```python
from build123d import *

# Parameters (mm, degrees)
BOSS_EXTRUDE1_DEPTH = 304.8
SHELL1_T            = -12.7


with BuildPart() as part:
    # Sketch1 → Boss-Extrude1 (new body)
    with BuildSketch(Plane(origin=(0, 0, 0), x_dir=(0, 0, -1), z_dir=(1, 0, 0))):
        Polygon((0, 0), (304.8, 0), (304.8, 56), (0, 109.74446372), align=None)
    extrude(amount=BOSS_EXTRUDE1_DEPTH)

    # Shell1
    shell1_openings = [part.faces().sort_by_distance(p)[0] for p in [
        (152.4, 82.87223186, -152.4),
    ]]
    offset(amount=SHELL1_T, openings=shell1_openings, kind=Kind.INTERSECTION)


solid = part.part
```
CAD build for the part. Positions are in the model's coordinates, mm. A direction names the side the tool comes from. Round coordinates to 2 decimals unless told otherwise and drop trailing zeros. Write each loop counter-clockwise with the first axis right and the second up, starting at its lowest first coordinate (ties: lowest second). Pieces come first, ordered by that corner, then holes. Notation, with made-up numbers: (32, 33.25) - (81, 33.25) arc R23 ccw to (81, 42.25) - close; hole circle Ø1 at (-34.5, -22.75). An arc over 180 degrees is marked (long way). Write item = value, one per line. Start each with the question number.
Q1. Band-saw the part on C-C (x = 219). Give the cut face in (y, z).
Q2. Band-saw the part on B-B (z = -130). Give the cut face in (x, y), then the cut area to 3 significant figures.
Q3. Band-saw the part on A-A (y = 20). Give the cut face in (x, z).
Q4. Which spindle directions (+Z, -Z, +X, -X, +Y, -Y) get a long thin tool onto all of the face, cutting with end or side? Do faces 1 (the flat face through (150, 61, -12.7)), 2 (the flat face through (150, 0, -150)). Say none if no direction does.
Q5. Drop flat-ended pins along their axis: pin 1 (3 mm diameter, centred on x = 140, z = -63.5, fed in from -Y); pin 2 (2 mm diameter, centred on x = 86.5, y = 76, fed in from -Z); pin 3 (5 mm diameter, centred on x = 39.5, z = -109.5, fed in from +Y). Give the stop position or say it passes through.
Q6. Mould opens along Z. For faces 3 (the flat face through (298.444, 80.756, -164.4)), 4 (the flat face through (150, 12.7, -150)), 5 (the flat face through (304.8, 43, -150)), 6 (the flat face through (292.1, 50, -150)) say: pulls with the +Z half, pulls with the -Z half, needs draft (parallel to the pull), parting line crosses it, or undercut.
Q7. Probe L1, parallel to X at y = 43.5, z = -53; L2, parallel to Z at x = 71, y = 39; L3, parallel to Y at x = 38, z = -279.5. List the from-to ranges inside material, lowest first. Write a range as from..to.
Answers below:
q1.outline = (0, -304.8) - (56, -304.8) - (58.24, -292.1) - (12.7, -292.1) - (12.7, -12.7) - (107.51, -12.7) - (109.74, 0) - (0, 0) - close
q2.outline = (0, 0) - (304.8, 0) - (304.8, 86.82) - (292.1, 86.82) - (292.1, 12.7) - (12.7, 12.7) - (12.7, 86.82) - (0, 86.82) - close
q2.area = 5,750 mm2
q3.outline = (0, -304.8) - (304.8, -304.8) - (304.8, 0) - (0, 0) - close; hole (12.7, -292.1) - (292.1, -292.1) - (292.1, -12.7) - (12.7, -12.7) - close
q4.face_1 = +Y
q4.face_2 = +Z, -Z, +X, -X, -Y
q5.pin_1 = 0
q5.pin_2 = -12.7
q5.pin_3 = 12.7
q6.face_3 = pulls with the -Z half
q6.face_4 = undercut
q6.face_5 = needs draft
q6.face_6 = undercut
q7.L1 = 0..12.7, 292.1..304.8
q7.L2 = -304.8..-292.1, -12.7..0
q7.L3 = 0..12.7
